For this review, use the dimensioned drawing (mm, ordinates from the lowest corner) and the shaded views. A direction names the side the tool comes from. Coordinates: 2 decimals unless noted, no trailing zeros. Order: outer loops, then holes, each group sorted by start corner. A loop starts at its lowest first (then second) coordinate and runs counter-clockwise, first axis right, second up. Notation, with made-up numbers: M 64.25,42.5 L 106.25,42.5 A30 cw 106.25,71.5 Z; hole C -34,74.25 d1. An arc over 180 degrees is marked long. One line per item, written item: value.
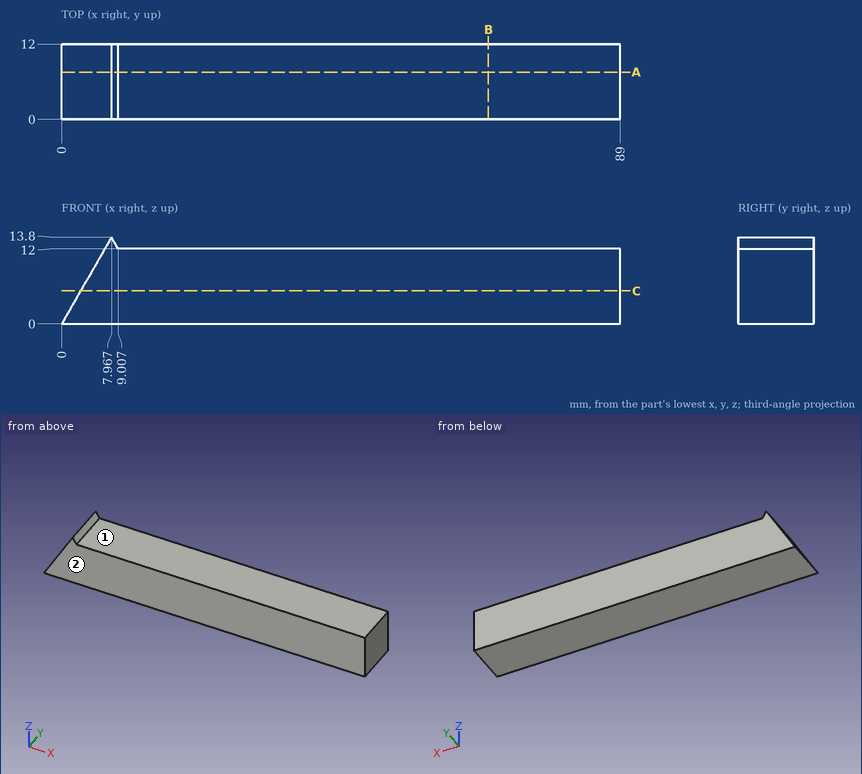
(1) We need section C-C, the plane z = 5.25. State the section outline as (x, y) points.
Geometry results:
outline: M 3.03,0 L 89,0 L 89,12 L 3.03,12 Z
(2) Tool access review of the marked faces 1 and 2: name each direction out of +Z, -Z, +X, -X, +Y, -Y from which nothing blocks a thin tool from reaching the whole face with its end or side.
Geometry results:
face 1: +Z, +X, +Y, -Y
face 2: +Z, -Z, +X, -X, -Y
(3) Insertion check: pin 1 Ø6 at (y, z) = (10, 7.5) entering from -X; pin 2 Ø2 at (x, y) = (23, 7) entering from +Z. Each pin has a flat end and moves straight along its axis. Give the tip position at first contact, or say it passes through.
Geometry results:
pin 1: stops at x = 2.6
pin 2: stops at z = 12
(4) For L1, parallel to Z at x = 57.5, y = 7.5; L2, parallel to X at y = 7, z = 12.75 (1 decimal); L3, parallel to X at y = 4, z = 9.75, list the stretches that pass through material, from the lowest coordinate up.
Geometry results:
L1: z = 0 to 12
L2: x = 7.4 to 8.6
L3: x = 5.63 to 89
(5) We need section B-B, the plane x = 68. State the section outline as (y, z) points.
Geometry results:
outline: M 0,0 L 12,0 L 12,12 L 0,12 Z
(6) We need section A-A, the plane y = 7.5. State the section outline as (x, z) points.
Geometry results:
outline: M 0,0 L 89,0 L 89,12 L 9.01,12 L 7.97,13.8 Z
